Design review of the part built by this model. Coordinates are the model's own, in mm. A direction names the side the tool comes from. Coordinates: 2 decimals unless noted, no trailing zeros. Write each loop counter-clockwise with the first axis right and the second up, starting at its lowest first coordinate (ties: lowest second). Pieces come first, ordered by that corner, then holes. Notation, with made-up numbers: M -23.5,-33.5 L 28.5,-33.5 A22 ccw 28.5,-9.5 Z; hole C 49,29.5 d11. An arc over 180 degrees is marked long. One line per question, with ' | ' between items.
from build123d import *

# Parameters (mm, degrees)
F0_W     = 56
F0_H     = 62
F1_DEPTH = 3
F2_R     = 3.25
F3_DEPTH = 3.5
F4_R     = 3.5
F5_W     = 21.484168
F5_H     = 37.344906
F6_DEPTH = 3.5


with BuildPart() as f1:
    # F0 (on Top) → F1 (new body)
    with BuildSketch(Plane.XY):
        with Locations((31.62972, 17.355853)):
            Rectangle(F0_W, F0_H)
    extrude(amount=F1_DEPTH)

    # F2 (on Top) → F3 (cut)
    with BuildSketch(Plane.XY):
        with Locations((52.62972, 42.855853)):
            Circle(F2_R)
        with Locations((10.62972, 42.855853)):
            Circle(F2_R)
    extrude(amount=F3_DEPTH, mode=Mode.SUBTRACT)

    # F4
    f4_edges = [f1.edges().sort_by_distance(p)[0] for p in [
        (3.62972, 48.355853, 1.5),
        (59.62972, 48.355853, 1.5),
    ]]
    fillet(f4_edges, radius=F4_R)

    # F5 (on face) → F6 (cut)
    with BuildSketch(Plane.XY.offset(3)):
        with Locations((31.681261, 14.266232)):
            Rectangle(F5_W, F5_H)
    extrude(amount=-F6_DEPTH, mode=Mode.SUBTRACT)


solid = f1.part
1. Insertion check: pin 1 Ø5 at (x, y) = (10.63, 42.86) entering from -Z. The pin has a flat end and moves straight along its axis. Give the tip position at first contact, or say it passes through.
Answer sheet:
pin 1: through
2. Take a section at B-B (x = 36). Write out the cut boundary in (y, z).
Answer sheet:
outline: M -13.64,0 L -4.41,0 L -4.41,3 L -13.64,3 Z; M 32.94,0 L 48.36,0 L 48.36,3 L 32.94,3 Z
3. To check wall thickness, follow line 1 along X through (y, z) = (19.5, 0.6); line 2 along Y through (x, z) = (28, 0.9); line 3 along X through (y, z) = (44, 1.4). State the ranges of each line that lie inside material, in increasing order. Write a range as [from, to].
Answer sheet:
line 1: [3.63, 20.94], [42.42, 59.63] | line 2: [-13.64, -4.41], [32.94, 48.36] | line 3: [3.63, 7.59], [13.67, 49.59], [55.67, 59.63]
4. Draft analysis for pull direction Y (two halves, no side actions). For faces 3 (the face through (50.05, 40.88, 1.48)), 4 (the face through (31, 48.356, 1)), 5 (the face through (59.63, 15, 1)), 6 (the face through (32, -4.406, 2)), state which applies: pulls with the +Y half, pulls with the -Y half, needs draft (parallel to the pull), parting line crosses it, or undercut.
Answer sheet:
face 3: undercut | face 4: pulls with the +Y half | face 5: needs draft | face 6: undercut
5. Take a section at A-A (y = 9). Write out the cut boundary in (x, z).
Answer sheet:
outline: M 3.63,0 L 20.94,0 L 20.94,3 L 3.63,3 Z; M 42.42,0 L 59.63,0 L 59.63,3 L 42.42,3 Z
6. Tool access review of faces 1 (the face through (44, 18, 3)), 2 (the face through (42.423, 14, 2)): name each direction out of +Z, -Z, +X, -X, +Y, -Y from which nothing blocks a thin tool from reaching the whole face with its end or side.
Answer sheet:
face 1: +Z, +X, -X, +Y, -Y | face 2: +Z, -Z
7. Take a section at C-C (z = 0.85). Write out the cut boundary in (x, y).
Answer sheet:
outline: M 3.63,-13.64 L 59.63,-13.64 L 59.63,44.86 A3.5 ccw 56.13,48.36 L 7.13,48.36 A3.5 ccw 3.63,44.86 Z; hole C 10.63,42.86 d6.5; hole M 20.94,-4.41 L 42.42,-4.41 L 42.42,32.94 L 20.94,32.94 Z; hole C 52.63,42.86 d6.5
